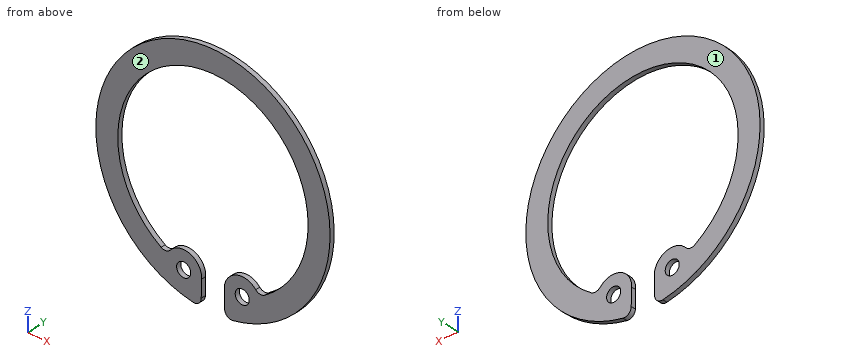
```python
from build123d import *

# Parameters (mm, degrees)
SKETCH1_R           = 12.7
SKETCH1_R_2         = 10.31875
BOSS_EXTRUDE1_DEPTH = 0.508
SKETCH2_W           = 2.54
SKETCH2_H           = 4.365272308
CUT_EXTRUDE1_DEPTH  = 0.508
FILLET1_R           = 0.762
BOSS_EXTRUDE2_START = -0.508
BOSS_EXTRUDE2_DEPTH = 0.508
SKETCH4_R           = 0.762
CUT_EXTRUDE2_DEPTH  = 0.508
CUT_EXTRUDE4_DEPTH  = 12.7
FILLET2_R           = 0.762
FILLET3_R           = 38.862


with BuildPart() as part:
    # Sketch1 → Boss-Extrude1 (new body)
    with BuildSketch(Plane(origin=(0, 0, 0), x_dir=(1, 0, 0), z_dir=(0, 1, 0))):
        with Locations(Location((0, 0, 0), (0, 0, 270))):
            Circle(SKETCH1_R)
        with Locations(Location((0, 0, 0), (0, 0, 270))):
            Circle(SKETCH1_R_2, mode=Mode.SUBTRACT)
    extrude(amount=BOSS_EXTRUDE1_DEPTH)

    # Sketch2 → Cut-Extrude1 (cut)
    with BuildSketch(Plane(origin=(0, 0.508, 0), x_dir=(1, 0, 0), z_dir=(0, 1, 0))):
        with Locations((0, 11.342245997)):
            Rectangle(SKETCH2_W, SKETCH2_H)
    extrude(amount=-CUT_EXTRUDE1_DEPTH, mode=Mode.SUBTRACT)

    # Fillet1
    fillet1_edges = [part.edges().sort_by_distance(p)[0] for p in [
        (-1.27, 0.254, -12.636340451),
        (1.27, 0.254, -12.636340451),
    ]]
    fillet(fillet1_edges, radius=FILLET1_R)

    # Sketch3 → Boss-Extrude2 (add)
    with BuildSketch(Plane(origin=(0, 0.508, 0), x_dir=(1, 0, 0), z_dir=(0, 1, 0)).offset(BOSS_EXTRUDE2_START)):
        with BuildLine():
            ThreePointArc((1.27, 10.240297924), (2.574626321, 7.9615922), (4.966472896, 9.044929438))
            ThreePointArc((4.966472896, 9.044929438), (3.175, 9.818145271), (1.27, 10.240297924))
        make_face()
    extrude(amount=BOSS_EXTRUDE2_DEPTH)

    # Sketch4 → Cut-Extrude2 (cut)
    with BuildSketch(Plane(origin=(0, 0.508, 0), x_dir=(-1, 0, 0), z_dir=(0, 1, 0))):
        with Locations(Location((-3.175, -9.818145271, 0), (0, 0, 90))):
            Circle(SKETCH4_R)
    extrude(amount=-CUT_EXTRUDE2_DEPTH, mode=Mode.SUBTRACT)

    # Sketch5 → Cut-Extrude4 (cut, symmetric)
    with BuildSketch(Plane(origin=(0, 0, 0), x_dir=(1, 0, 0), z_dir=(0, 1, 0))):
        Polygon((0, 13.122692647), (0, -13.667441161), (-16.637303015, -10.48078624), (-17.785980951, 10.084254234), (-7.744312539, 13.715558678), align=None)
    extrude(amount=CUT_EXTRUDE4_DEPTH, both=True, mode=Mode.SUBTRACT)

    # Fillet2
    fillet2_edges = [part.edges().sort_by_distance(p)[0] for p in [
        (4.966472896, 0.254, -9.044929438),
    ]]
    fillet(fillet2_edges, radius=FILLET2_R)

    # Fillet3
    fillet3_edges = [part.edges().sort_by_distance(p)[0] for p in [
        (1.27, 0.254, -10.240297924),
    ]]
    fillet(fillet3_edges, radius=FILLET3_R)

    # Mirror1: part across plane


with BuildPart() as part_1:
    add(part.part)
    add(part.part.mirror(Plane(origin=(0, 0, 0), x_dir=(0, 0, 1), z_dir=(1, 0, 0))))


solid = part_1.part
```
CAD build for the part. Positions are in the model's coordinates, mm. Face numbers are marked on the shaded views. Give positions to 0.01 mm unless a question says otherwise; leave off trailing zeros. Loops run counter-clockwise (first coordinate to the right, second up) from the corner with the lowest first, then second, coordinate; pieces in that order, holes last. Notation, with made-up numbers: (71, -16.75) -> (92, -16.75) arc R10 cw to (92, -8.75) -> close; hole circle Ø7 at (75, 2.25). An arc over 180 degrees is marked (long way). Use a Markdown table: item, result.
1. Slice it at A-A (z = 0). List the corners of the cut face in (x, y), plus the area to 3 significant figures.
Check result:
| item | result |
|---|---|
| outline | (-12.7, 0) -> (-10.32, 0) -> (-10.32, 0.51) -> (-12.7, 0.51) -> close; (10.32, 0) -> (12.7, 0) -> (12.7, 0.51) -> (10.32, 0.51) -> close |
| area | 2.42 mm^2 |
2. Wall check: L1, parallel to X at y = 0.25, z = 0; L2, parallel to Z at x = 0, y = 0.25; L3, parallel to X at y = 0.1, z = -8.25. Give the ranges that are in metal, low to high. Write a range as [from, to].
Check result:
| item | result |
|---|---|
| L1 | x = [-12.7, -10.32], [10.32, 12.7] |
| L2 | z = [10.32, 12.7] |
| L3 | x = [-9.66, -6.2], [-4.34, -2.01], [2.01, 4.34], [6.2, 9.66] |
3. Slice it at D-D (y = 0.35). Give the number of separate pieces and of enclosed holes in the cut face, plus the area to 3 significant figures.
Check result:
| item | result |
|---|---|
| separate pieces | 1 |
| enclosed holes | 2 |
| area | 174 mm^2 |
4. Flat gauge pin, fed straight in: pin 1 (10 mm diameter, centred on x = -2, z = 0.5, fed in from -Y). Where does the tip first touch, or does it go through?
Check result:
| item | result |
|---|---|
| pin 1 | passes through |
5. Slice it at B-B (x = -10). List the corners of the cut face in (y, z), plus the area to 3 significant figures.
Check result:
| item | result |
|---|---|
| outline | (0, -7.83) -> (0.51, -7.83) -> (0.51, -2.54) -> (0, -2.54) -> close; (0, 2.54) -> (0.51, 2.54) -> (0.51, 7.83) -> (0, 7.83) -> close |
| area | 5.37 mm^2 |
6. Mould opens along Y. For the marked faces 1 and 2 say: pulls with the +Y half, pulls with the -Y half, needs draft (parallel to the pull), parting line crosses it, or undercut.
Check result:
| item | result |
|---|---|
| face 1 | pulls with the +Y half |
| face 2 | pulls with the -Y half |
7. Slice it at C-C (x = 0). List the corners of the cut face in (y, z).
Check result:
| item | result |
|---|---|
| outline | (0, 10.32) -> (0.51, 10.32) -> (0.51, 12.7) -> (0, 12.7) -> close |
